CAD build for the part. Positions are in the model's coordinates, mm. A direction names the side the tool comes from. Coordinates: 2 decimals unless noted, no trailing zeros. Loops run counter-clockwise (first coordinate to the right, second up) from the corner with the lowest first, then second, coordinate; pieces in that order, holes last. Notation, with made-up numbers: (-8, 10.5) -> (-3, 10.5) arc R31 cw to (-3, 45.5) -> close; hole circle Ø8 at (-21.5, -16). An arc over 180 degrees is marked (long way). Return JSON: item names as keys, results as strings. Group by question number.
(1) Tool access for faces 1 (the face through (40, 0, -13)), 2 (the face through (12, 2, -10)): list every direction of +Z, -Z, +X, -X, +Y, -Y with a clear straight run to the whole face (end or side of a thin tool).
(2) Probe L1, parallel to Z at x = 40.5, y = 1.4; L2, parallel to Z at x = 68.5, y = 1.6; L3, parallel to Y at x = 9, z = -2.5. List the from-to ranges inside material, lowest first.
(3) Saw through at B-B on x = 40.5. Write the cut outline in (y, z), then the cut area to 3 significant figures.
(4) Mould opens along X. For faces 3 (the face through (81, 11, -10)), 4 (the face through (40, 2, -10)), 5 (the face through (0, 11, -10)), 6 (the face through (40, 8, 0)) say: pulls with the +X half, pulls with the -X half, needs draft (parallel to the pull), parting line crosses it, or undercut.
(5) Saw through at A-A on x = 12.5. Write the cut outline in (y, z), then the cut area to 3 significant figures.
(6) Saw through at C-C on y = 19. Write the cut outline in (x, z).
(7) Flat gauge pins, fed straight in: pin 1 Ø0.8 at (x, z) = (41, -10) entering from -Y; pin 2 Ø3 at (x, z) = (32.5, -18.5) entering from +Y; pin 3 Ø8 at (y, z) = (14.5, -18) entering from -X. Where does each tip first touch, or does it go through?
Autodesk Inventor part; units mm, degrees
ref_plane "YZ Plane" through (0, 0, 0) normal (1, 0, 0) x (0, 1, 0)
ref_plane "XZ Plane" through (0, 0, 0) normal (0, 1, 0) x (-1, 0, 0)
ref_plane "XY Plane" through (0, 0, 0) normal (0, 0, 1) x (1, 0, 0)
sketch "스케치1" plane through (0, 0, 0) normal (1, 0, 0) x (0, 1, 0)
  line L0 (0, 0) -> (21.5, 0)
  line L1 (21.5, 0) -> (21.5, -21)
  line L2 (21.5, -21) -> (0, -21)
  line L3 (0, -21) -> (0, 0)
  dimension "d0" = 21.5
  dimension "d1" = 21
extrude "돌출1" add sketch "스케치1" along normal blind 81
fillet "모깎기1" radius 5 2 edges at (40.5, 21.5, 0) (40.5, 21.5, -21)
sketch "스케치2" plane through (0, 0, -21) normal (0, -1, 0) x (1, 0, 0)
  point P0 (0, 21)
sketch "스케치3" plane through (0, 0, -21) normal (0, -1, 0) x (1, 0, 0)
  line L0 (0, 0) -> (81, 0)
  line L1 (40.5, 0) -> (40.5, 10.5)
  line L2 (0, 21) -> (81, 21)
  circle A0 centre (40.5, 10.5) radius 1.25
  line L3 (40.5, 10.5) -> (68.5, 10.5)
  circle A1 centre (68.5, 10.5) radius 1.5
  line L4 (40.5, 10.5) -> (12.5, 10.5)
  circle A2 centre (12.5, 10.5) radius 1.5
  dimension "d5" = 10.5
  dimension "d6" = 2.5
  dimension "d7" = 28
  dimension "d8" = 3
  dimension "d9" = 28
  dimension "d10" = 3
extrude "돌출2" cut sketch "스케치3" against normal blind 2
properties part number "배터리+홀더"
Geometry results:
{
 "1": {"face 1": "+Z, -Z, +X, -X, -Y", "face 2": "-Y"},
 "2": {"L1": "-21 to -11.75, -9.25 to 0", "L2": "-21 to -12, -9 to 0", "L3": "0 to 20.83"},
 "3": {"outline": "(0, -21) -> (16.5, -21) arc R5 ccw to (21.5, -16) -> (21.5, -5) arc R5 ccw to (16.5, 0) -> (0, 0) -> (0, -9.25) -> (2, -9.25) -> (2, -11.75) -> (0, -11.75) -> close", "area": "436 mm²"},
 "4": {"face 3": "pulls with the +X half", "face 4": "undercut", "face 5": "pulls with the -X half", "face 6": "needs draft"},
 "5": {"outline": "(0, -21) -> (16.5, -21) arc R5 ccw to (21.5, -16) -> (21.5, -5) arc R5 ccw to (16.5, 0) -> (0, 0) -> (0, -9) -> (2, -9) -> (2, -12) -> (0, -12) -> close", "area": "435 mm²"},
 "6": {"outline": "(0, -20.33) -> (81, -20.33) -> (81, -0.67) -> (0, -0.67) -> close"},
 "7": {"pin 1": "y = 2", "pin 2": "y = 21.4", "pin 3": "x = 0"}
}
